The listing builds one solid part. Answer for the finished solid, in the listing's coordinates (mm). A direction names the side the tool comes from. Give positions to 0.01 mm unless a question says otherwise; leave off trailing zeros. Order: outer loops, then holes, each group sorted by start corner. A loop starts at its lowest first (then second) coordinate and runs counter-clockwise, first axis right, second up.
```python
from build123d import *

# Parameters (mm, degrees)
SKETCH1_W           = 42
SKETCH1_H           = 42
BOSS_EXTRUDE1_DEPTH = 2
SKETCH2_R           = 11.5
CUT_EXTRUDE1_DEPTH  = 30.765752132
SKETCH3_R           = 2
CUT_EXTRUDE2_DEPTH  = 30.765752132
CUT_EXTRUDE3_DEPTH  = 30.765752132
SKETCH5_W           = 2
SKETCH5_H           = 32.100505064
BOSS_EXTRUDE2_DEPTH = 10
SKETCH6_W           = 5
SKETCH6_H           = 5
BOSS_EXTRUDE3_DEPTH = 10
SKETCH9_W           = 4
SKETCH9_H           = 12
CUT_EXTRUDE4_DEPTH  = 1
SKETCH11_R          = 1.5
CUT_EXTRUDE5_DEPTH  = 4
FILLET1_R           = 2


with BuildPart() as part:
    # Sketch1 → Boss-Extrude1 (new body)
    with BuildSketch(Plane(origin=(0, 0, 0), x_dir=(1, 0, 0), z_dir=(0, 1, 0))):
        Rectangle(SKETCH1_W, SKETCH1_H)
    extrude(amount=BOSS_EXTRUDE1_DEPTH)

    # Sketch2 → Cut-Extrude1 (cut, through all)
    with BuildSketch(Plane(origin=(0, 2, 0), x_dir=(1, 0, 0), z_dir=(0, 1, 0))):
        with Locations(Location((0, 0, 0), (0, 0, 270))):
            Circle(SKETCH2_R)
    extrude(amount=-CUT_EXTRUDE1_DEPTH, mode=Mode.SUBTRACT)

    # Sketch3 → Cut-Extrude2 (cut, through all)
    with BuildSketch(Plane(origin=(0, 2, 0), x_dir=(1, 0, 0), z_dir=(0, 1, 0))):
        with Locations(Location((-15.5, 15.5, 0), (0, 0, 270))):
            Circle(SKETCH3_R)
        with Locations(Location((15.5, 15.5, 0), (0, 0, 270))):
            Circle(SKETCH3_R)
        with Locations(Location((15.5, -15.5, 0), (0, 0, 270))):
            Circle(SKETCH3_R)
        with Locations(Location((-15.5, -15.5, 0), (0, 0, 270))):
            Circle(SKETCH3_R)
    extrude(amount=-CUT_EXTRUDE2_DEPTH, mode=Mode.SUBTRACT)

    # Sketch4 → Cut-Extrude3 (cut, through all)
    with BuildSketch(Plane(origin=(0, 2, 0), x_dir=(1, 0, 0), z_dir=(0, 1, 0))):
        Polygon((-21, 16.050252532), (-16.050252532, 21), (-21, 21), align=None)
        Polygon((-21, -21), (-16.050252532, -21), (-21, -16.050252532), align=None)
        Polygon((21, -21), (16.050252532, -21), (21, -16.050252532), align=None)
        Polygon((16.050252532, 21), (21, 16.050252532), (21, 21), align=None)
    extrude(amount=-CUT_EXTRUDE3_DEPTH, mode=Mode.SUBTRACT)

    # Sketch5 → Boss-Extrude2 (add)
    with BuildSketch(Plane(origin=(0, 2, 0), x_dir=(1, 0, 0), z_dir=(0, 1, 0))):
        with Locations((-20, 0)):
            Rectangle(SKETCH5_W, SKETCH5_H)
        with Locations((20, 0)):
            Rectangle(SKETCH5_W, SKETCH5_H)
    extrude(amount=BOSS_EXTRUDE2_DEPTH)

    # Sketch6 → Boss-Extrude3 (add)
    with BuildSketch(Plane(origin=(0, 2, 0), x_dir=(1, 0, 0), z_dir=(0, 1, 0))):
        with Locations((6.5, -15.5)):
            Rectangle(SKETCH6_W, SKETCH6_H)
        with Locations((-6.5, 15.5)):
            Rectangle(SKETCH6_W, SKETCH6_H)
    extrude(amount=BOSS_EXTRUDE3_DEPTH)

    # Sketch9 → Cut-Extrude4 (cut)
    with BuildSketch(Plane(origin=(21, 0, 0), x_dir=(0, 0, -1), z_dir=(1, 0, 0))):
        with Locations((0, 6)):
            Rectangle(SKETCH9_W, SKETCH9_H)
    extrude(amount=-CUT_EXTRUDE4_DEPTH, mode=Mode.SUBTRACT)

    # Sketch11 → Cut-Extrude5 (cut)
    with BuildSketch(Plane(origin=(0, 12, 0), x_dir=(1, 0, 0), z_dir=(0, 1, 0))):
        with Locations(Location((-6.5, 15.474657956, 0), (0, 0, 270))):
            Circle(SKETCH11_R)
        with Locations(Location((6.5, -15.5, 0), (0, 0, 270))):
            Circle(SKETCH11_R)
    extrude(amount=-CUT_EXTRUDE5_DEPTH, mode=Mode.SUBTRACT)

    # Fillet1
    fillet1_edges = [part.edges().sort_by_distance(p)[0] for p in [
        (9, 7, 18),
        (9, 7, 13),
        (-9, 7, -18),
        (-9, 7, -13),
    ]]
    fillet(fillet1_edges, radius=FILLET1_R)


solid = part.part
```
1) Given P1, Ø4.5, axis at x = 15.5, z = 15.5, coming from the +Y side; P2, Ø2, axis at x = -20, y = 5, coming from the -Z side; P3, Ø0.6, axis at x = 20.5, y = 6, coming from the +Z side, each flat-ended and moving along its own axis, determine where each tip first touches the part or whether it passes through.
Geometry says:
P1: stops at y = 2
P2: stops at z = -16.05
P3: stops at z = 16.05
2) Find section B-B (z = 0). Write down the section's boundary in (x, y), then the cut area to 3 significant figures.
Geometry says:
outline: (-21, 0) - (-11.5, 0) - (-11.5, 2) - (-19, 2) - (-19, 12) - (-21, 12) - close; (11.5, 0) - (20, 0) - (20, 12) - (19, 12) - (19, 2) - (11.5, 2) - close
area: 66.0 mm2
3) Straight lines are drawn through the part: probe 1 along X at (y, z) = (1.25, 15.5); probe 2 along X at (y, z) = (3.5, 6); probe 3 along X at (y, z) = (9, -16) (3 decimals). For each, find the intervals that lie inside material, in ascending order.
Geometry says:
probe 1: x = -21 to -17.5, -13.5 to 13.5, 17.5 to 21
probe 2: x = -21 to -19, 19 to 21
probe 3: x = -21 to -19, -9 to -7.905, -5.095 to -4, 19 to 21
4) Find section A-A (y = 11.25). Write down the section's boundary in (x, z), then the cut area to 3 significant figures.
Geometry says:
outline: (-21, -16.05) - (-19, -16.05) - (-19, 16.05) - (-21, 16.05) - close; (-9, -16) arc R2 ccw to (-7, -18) - (-4, -18) - (-4, -13) - (-7, -13) arc R2 ccw to (-9, -15) - close; (4, 13) - (7, 13) arc R2 ccw to (9, 15) - (9, 16) arc R2 ccw to (7, 18) - (4, 18) - close; (19, -16.05) - (21, -16.05) - (21, -2) - (20, -2) - (20, 2) - (21, 2) - (21, 16.05) - (19, 16.05) - close; hole circle Ø3 at (-6.5, -15.47); hole circle Ø3 at (6.5, 15.5)
area: 157 mm2
5) Find section D-D (x = 0). Write down the section's boundary in (y, z), then the cut area to 3 significant figures.
Geometry says:
outline: (0, -21) - (2, -21) - (2, -11.5) - (0, -11.5) - close; (0, 11.5) - (2, 11.5) - (2, 21) - (0, 21) - close
area: 38.0 mm2
6) Find section C-C (y = 6.25). Write down the section's boundary in (x, z), then the cut area to 3 significant figures.
Geometry says:
outline: (-21, -16.05) - (-19, -16.05) - (-19, 16.05) - (-21, 16.05) - close; (-9, -16) arc R2 ccw to (-7, -18) - (-4, -18) - (-4, -13) - (-7, -13) arc R2 ccw to (-9, -15) - close; (4, 13) - (7, 13) arc R2 ccw to (9, 15) - (9, 16) arc R2 ccw to (7, 18) - (4, 18) - close; (19, -16.05) - (21, -16.05) - (21, -2) - (20, -2) - (20, 2) - (21, 2) - (21, 16.05) - (19, 16.05) - close
area: 171 mm2
7) For a pull along Z with two mould halves and no side action, classify faces 1 (the flat face through (-20, 7, 16.05)), 2 (the flat face through (20.5, 5.9, -2)), 3 (the flat face through (21, 6, -9)) as +Z half, -Z half, draft (parallel to the pull), parting line (faces both ways), or undercut.
Geometry says:
face 1: +Z half
face 2: undercut
face 3: draft
8) A tool of negligible diameter and unlimited length cuts with its end or side. For faces 4 (the flat face through (7, 8, 15)), 5 (the flat face through (4, 7, 16)), 6 (the flat face through (-20, 7, -16.05)), from which of +Z, -Z, +X, -X, +Y, -Y can it reach the whole face along a straight path? Write none if from no direction.
Geometry says:
face 4: +Y
face 5: +Z, -Z, +Y
face 6: -Z, -X, +Y
